Geometry: final body of the model. Coordinates: model frame, mm. A direction names the side the tool comes from. Coordinates: 2 decimals unless noted, no trailing zeros. Order: outer loops, then holes, each group sorted by start corner. A loop starts at its lowest first (then second) coordinate and runs counter-clockwise, first axis right, second up. Notation, with made-up numbers: (81.25, 86) -> (138.25, 86) arc R17 ccw to (138.25, 111) -> close; hole circle Ø9 at (59.25, -20.75). An arc over 180 degrees is marked (long way). Answer in a Markdown table with one row per item. Add a question column.
1) Contact query for flat-ended pins moving along their axis: P1, Ø10, axis at x = -38, y = 28.5, coming from the +Z side; P2, Ø15.5, axis at x = -72, z = 48.5, coming from the +Y side; P3, Ø13.5, axis at x = 54, y = 82.7, coming from the -Z side; P4, Ø5, axis at x = -12.5, y = 201, coming from the -Z side. Output: stop coordinate, or through.
2) Section query D-D on y = 110.5. Return the cut outline in (x, z).
3) Section query A-A on x = 54. Return the cut outline in (y, z).
4) Ray query, line 1 (Y direction, x = 54, z = 5); line 2 (Y direction, x = 0, z = -13.5); line 3 (Y direction, x = 0, z = 3). Return the intervals inside material, ascending. Write a range as from..to.
5) Section query C-C on y = 74. Return the cut outline in (x, z).
6) Set-up query: faces 4 (the face through (-10.84, 89.65, -17.6)), 5 (the face through (-5, 4.5, 0)), 6 (the face through (9.69, 91.87, 17.6)). Return all of +Z, -Z, +X, -X, +Y, -Y with unobstructed straight access to the full face (end or side cutting, diameter ignored); none if empty.
7) Section query B-B on z = 49.15. Return the cut outline in (x, y).
8) Pull-direction query (Y, two-part tool) for faces 1 (the face through (-62, 63, 55)), 2 (the face through (-62, 78.5, 25)), 3 (the face through (-62, 48.5, 25)); classes: +Y half, -Y half, draft (parallel to the pull), parting line (faces both ways), or undercut.
```python
from build123d import *

# Parameters (mm, degrees)
SKETCH1_W                         = 75
SKETCH1_H                         = 50
BE_MAIN_UPRIGHT_BODY_DEPTH        = 221
SKETCH4_R                         = 12.5
CE_THROUGH_HOLE_DEPTH             = 230.667694724
SKETCH2_R                         = 21
CE_INNER_BEARING_DEPTH            = 15
SKETCH3_R                         = 23.5
CE_OUTER_BEARING_DEPTH            = 15
SKETCH7_W                         = 26.55070312
SKETCH7_H                         = 111.194580496
BE_CALIPER_MOUNT_DEPTH            = 33
SKETCH8_W                         = 21.441072272
SKETCH8_H                         = 20
BE_TEMP_SENSOR_MOUNT_DEPTH        = 50
SKETCH9_W                         = 60
SKETCH9_H                         = 30
BE_TIE_ROD_MOUNT_DEPTH            = 50
SKETCH10_R                        = 5.968024458
CE_CALIPER_HOLES_DEPTH            = 242.325913005
SKETCH12_R                        = 4
CE_TOP_CLEVIS_HOLES_DEPTH         = 243.893495178
SKETCH13_W                        = 55
SKETCH13_H                        = 20
CE_TOP_CLEVIS_SPACE_DEPTH         = 35
SKETCH14_W                        = 25
SKETCH14_H                        = 12
CE_BOTTOM_CLEVIS_SPACE_DEPTH      = 243.893495178
SKETCH15_W                        = 25
SKETCH15_H                        = 5
CE_EXPAND_BOTTOM_CLEVIS_DEPTH     = 243.893495178
CE_WIDEN_BOTTOM_CLEVIS_DEPTH      = 240.74121548
CE_WIDEN_BOTTOM_CLEVIS_DEPTH_BACK = 240.74121548
SKETCH16_W                        = 10.007554032
SKETCH16_H                        = 17
CHAMFER1_SIZE                     = 30
SKETCH18_W                        = 14.04398123
SKETCH18_H                        = 13.562779604
CUT_EXTRUDE1_DEPTH                = 20
SKETCH19_R                        = 3
CUT_EXTRUDE2_DEPTH                = 177.032667423
SKETCH20_R                        = 4
CUT_EXTRUDE3_DEPTH                = 242.780729009


with BuildPart() as part:
    # Sketch1 → BE - main upright body (new body)
    with BuildSketch(Plane(origin=(0, 0, 0), x_dir=(1, 0, 0), z_dir=(0, 1, 0))):
        Rectangle(SKETCH1_W, SKETCH1_H)
    extrude(amount=BE_MAIN_UPRIGHT_BODY_DEPTH)

    # Sketch4 → CE - Through hole (cut, through all)
    with BuildSketch(Plane.XY.offset(25)):
        with Locations((0, 110.5)):
            Circle(SKETCH4_R)
    extrude(amount=-CE_THROUGH_HOLE_DEPTH, mode=Mode.SUBTRACT)

    # Sketch2 → CE - Inner bearing (cut)
    with BuildSketch(Plane.XY.offset(25)):
        with Locations((0, 110.5)):
            Circle(SKETCH2_R)
    extrude(amount=-CE_INNER_BEARING_DEPTH, mode=Mode.SUBTRACT)

    # Sketch3 → CE - Outer bearing (cut)
    with BuildSketch(Plane(origin=(0, 0, -25), x_dir=(-1, 0, 0), z_dir=(0, 0, -1))):
        with Locations((0, 110.5)):
            Circle(SKETCH3_R)
    extrude(amount=-CE_OUTER_BEARING_DEPTH, mode=Mode.SUBTRACT)

    # Sketch7 → BE - caliper mount (add)
    with BuildSketch(Plane(origin=(37.5, 0, 0), x_dir=(0, 0, -1), z_dir=(1, 0, 0))):
        with Locations((0, 110.5)):
            Rectangle(SKETCH7_W, SKETCH7_H)
    extrude(amount=BE_CALIPER_MOUNT_DEPTH)

    # Sketch8 → BE - temp sensor mount (add)
    with BuildSketch(Plane.ZY.offset(37.5)):
        with Locations((0, 148.452249223)):
            Rectangle(SKETCH8_W, SKETCH8_H)
    extrude(amount=BE_TEMP_SENSOR_MOUNT_DEPTH)

    # Sketch9 → BE - tie rod mount (add)
    with BuildSketch(Plane.ZY.offset(37.5)):
        with Locations((25, 63.5)):
            Rectangle(SKETCH9_W, SKETCH9_H)
    extrude(amount=BE_TIE_ROD_MOUNT_DEPTH)

    # Sketch10 → CE - caliper holes (cut, through all)
    with BuildSketch(Plane.XY.offset(13.27535156)):
        with Locations((54, 138.298645124)):
            Circle(SKETCH10_R)
        with Locations((54, 82.701354876)):
            Circle(SKETCH10_R)
    extrude(amount=-CE_CALIPER_HOLES_DEPTH, mode=Mode.SUBTRACT)

    # Sketch12 → CE - top clevis holes (cut, through all)
    with BuildSketch(Plane.XY.offset(25)):
        with Locations((-12.5, 201)):
            Circle(SKETCH12_R)
        with Locations((12.5, 201)):
            Circle(SKETCH12_R)
    extrude(amount=-CE_TOP_CLEVIS_HOLES_DEPTH, mode=Mode.SUBTRACT)

    # Sketch13 → CE - top clevis space (cut)
    with BuildSketch(Plane.XY.offset(25)):
        with Locations((0, 201)):
            Rectangle(SKETCH13_W, SKETCH13_H)
    extrude(amount=-CE_TOP_CLEVIS_SPACE_DEPTH, mode=Mode.SUBTRACT)

    # Sketch14 → CE - bottom clevis space (cut, through all)
    with BuildSketch(Plane.XY.offset(25)):
        with Locations((-9.98, 10.5)):
            Rectangle(SKETCH14_W, SKETCH14_H)
    extrude(amount=-CE_BOTTOM_CLEVIS_SPACE_DEPTH, mode=Mode.SUBTRACT)

    # Sketch15 → CE - expand bottom clevis (cut, through all)
    with BuildSketch(Plane.XY.offset(25)):
        with Locations((-9.98, 19)):
            Rectangle(SKETCH15_W, SKETCH15_H)
    extrude(amount=-CE_EXPAND_BOTTOM_CLEVIS_DEPTH, mode=Mode.SUBTRACT)

    # Sketch16 → CE - widen bottom clevis (cut, two sides: drawn at the far end of the back side and taken through both)
    with BuildSketch(Plane(origin=(2.52, 4.5, 25), x_dir=(1, 0, 0), z_dir=(0, 0, 1)).offset(-CE_WIDEN_BOTTOM_CLEVIS_DEPTH_BACK)):
        with Locations((5.003777016, 8.5)):
            Rectangle(SKETCH16_W, SKETCH16_H)
    extrude(amount=CE_WIDEN_BOTTOM_CLEVIS_DEPTH + CE_WIDEN_BOTTOM_CLEVIS_DEPTH_BACK, mode=Mode.SUBTRACT)

    # Chamfer1
    chamfer1_edges = [part.edges().sort_by_distance(p)[0] for p in [
        (-87.5, 63.5, -5),
    ]]
    chamfer(chamfer1_edges, length=CHAMFER1_SIZE)

    # Sketch18 → Cut-Extrude1 (cut)
    with BuildSketch(Plane.XY.offset(55)):
        with Locations((-73.48, 63.84)):
            Rectangle(SKETCH18_W, SKETCH18_H)
    extrude(amount=-CUT_EXTRUDE1_DEPTH, mode=Mode.SUBTRACT)

    # Sketch19 → Cut-Extrude2 (cut, through all)
    with BuildSketch(Plane(origin=(0, 78.5, 0), x_dir=(1, 0, 0), z_dir=(0, 1, 0))):
        with Locations(Location((-73.48, -49.15, 0), (0, 0, 270))):
            Circle(SKETCH19_R)
    extrude(amount=-CUT_EXTRUDE2_DEPTH, mode=Mode.SUBTRACT)

    # Sketch20 → Cut-Extrude3 (cut, through all)
    with BuildSketch(Plane.XY.offset(10.720536136)):
        with Locations((-53.502606246, 148.452249223)):
            Circle(SKETCH20_R)
        with Locations((-71.497393754, 148.452249223)):
            Circle(SKETCH20_R)
    extrude(amount=-CUT_EXTRUDE3_DEPTH, mode=Mode.SUBTRACT)


solid = part.part
```
Result:
| question | item | result |
|---|---|---|
| 1 | P1 | z = 25 |
| 1 | P2 | y = 78.5 |
| 1 | P3 | z = -13.28 |
| 1 | P4 | through |
| 2 | outline | (-37.5, -25) -> (-23.5, -25) -> (-23.5, -10) -> (-12.5, -10) -> (-12.5, 10) -> (-21, 10) -> (-21, 25) -> (-37.5, 25) -> close; (12.5, -10) -> (23.5, -10) -> (23.5, -25) -> (37.5, -25) -> (37.5, -13.28) -> (70.5, -13.28) -> (70.5, 13.28) -> (37.5, 13.28) -> (37.5, 25) -> (21, 25) -> (21, 10) -> (12.5, 10) -> close |
| 3 | outline | (54.9, -13.28) -> (76.73, -13.28) -> (76.73, 13.28) -> (54.9, 13.28) -> close; (88.67, -13.28) -> (132.33, -13.28) -> (132.33, 13.28) -> (88.67, 13.28) -> close; (144.27, -13.28) -> (166.1, -13.28) -> (166.1, 13.28) -> (144.27, 13.28) -> close |
| 4 | line 1 | 54.9..76.73, 88.67..132.33, 144.27..166.1 |
| 4 | line 2 | 0..4.5, 21.5..87, 134..221 |
| 4 | line 3 | 0..4.5, 21.5..98, 123..191, 211..221 |
| 5 | outline | (-87.5, 25) -> (-57.5, -5) -> (-37.5, -5) -> (-37.5, -25) -> (37.5, -25) -> (37.5, -13.28) -> (70.5, -13.28) -> (70.5, 13.28) -> (37.5, 13.28) -> (37.5, 25) -> (-37.5, 25) -> (-37.5, 55) -> (-87.5, 55) -> close; hole circle Ø6 at (-73.48, 49.15) |
| 6 | face 4 | -Z |
| 6 | face 5 | +Z, -Z |
| 6 | face 6 | +Z |
| 7 | outline | (-87.5, 48.5) -> (-76.48, 48.5) -> (-76.48, 57.06) -> (-80.5, 57.06) -> (-80.5, 70.62) -> (-76.48, 70.62) -> (-76.48, 78.5) -> (-87.5, 78.5) -> close; (-70.48, 48.5) -> (-37.5, 48.5) -> (-37.5, 78.5) -> (-70.48, 78.5) -> (-70.48, 70.62) -> (-66.46, 70.62) -> (-66.46, 57.06) -> (-70.48, 57.06) -> close |
| 8 | face 1 | draft |
| 8 | face 2 | undercut |
| 8 | face 3 | -Y half |
